Autodesk Fusion 360 part; units mm, degrees
sketch "Sketch1" plane through (0, 0, 0) normal (0, 0, 1) x (1, 0, 0)
  line L0 (0, 0) -> (50.8, 0)
  line L1 (50.8, 0) -> (50.8, 50.8)
  line L2 (50.8, 50.8) -> (0, 50.8)
  line L3 (0, 50.8) -> (0, 0)
  dimension "d1" = 50.8
  dimension "d2" = 50.8
extrude "Extrude1" add sketch "Sketch1" along normal blind 31.75
sketch "Sketch2" plane through (50.8, 0, 0) normal (1, 0, 0) x (0, 1, 0)
  line L0 (0, 0) -> (50.8, 0)
  line L1 (50.8, 0) -> (50.8, 31.75)
  line L2 (50.8, 31.75) -> (0, 31.75)
  line L3 (0, 31.75) -> (0, 0)
  line L4 (50.8, 23.368) -> (10.16, 23.368)
  line L5 (10.16, 23.368) -> (10.16, 3.81)
  line L6 (10.16, 3.81) -> (50.8, 3.81)
  line L7 (50.8, 3.81) -> (50.8, 23.368)
  dimension "d5" = 40.64
  dimension "d6" = 19.558
  dimension "d14" = 3.81
extrude "Extrude2" cut sketch "Sketch2" against normal blind 40.64 contours L1 L4 L5 L6 L7
sketch "Sketch3" plane through (0, 0, 31.75) normal (0, 0, 1) x (-1, 0, 0)
  line L0 (0, -50.8) -> (0, 0)
  line L1 (0, 0) -> (-50.8, 0)
  line L2 (-50.8, 0) -> (-50.8, -50.8)
  line L3 (-50.8, -50.8) -> (0, -50.8)
  line L4 (0, 0) -> (-25.4, 0)
  line L5 (-25.4, 0) -> (-25.4, -25.4)
  line L6 (-25.4, -25.4) -> (0, -25.4)
  line L7 (0, -25.4) -> (0, 0)
  dimension "d10" = 25.4
  dimension "d11" = 25.4
extrude "Extrude3" add sketch "Sketch3" along normal blind 152.4 contours L0 L1 L4 L5 L6 L7
fillet "Fillet1" radius 2.54 2 edges at (25.4, 12.7, 31.75) (12.7, 25.4, 31.75)
sketch "Sketch4" plane through (0, 0, 0) normal (0, 0, -1) x (1, 0, 0)
  line L0 (0, 0) -> (0, -50.8)
  line L1 (0, -50.8) -> (50.8, -50.8)
  line L2 (50.8, -50.8) -> (50.8, 0)
  line L3 (50.8, 0) -> (0, 0)
  line L4 (2.54, -2.54) -> (22.86, -2.54)
  line L5 (22.86, -2.54) -> (22.86, -22.86)
  line L6 (22.86, -22.86) -> (2.54, -22.86)
  line L7 (2.54, -22.86) -> (2.54, -2.54)
  dimension "d17" = 2.54
  dimension "d18" = 2.54
  dimension "d19" = 20.32
  dimension "d20" = 20.32
sketch "Sketch5" plane through (0, 0, 0) normal (0, 0, -1) x (1, 0, 0)
  line L0 (5.08, -5.08) -> (20.32, -5.08)
  line L1 (20.32, -5.08) -> (20.32, -20.32)
  line L2 (20.32, -20.32) -> (5.08, -20.32)
  line L3 (5.08, -20.32) -> (5.08, -5.08)
  line L4 (2.54, -2.54) -> (22.86, -2.54)
  line L5 (2.54, -22.86) -> (2.54, -2.54)
  dimension "d21" = 2.54
  dimension "d22" = 2.54
  dimension "d23" = 15.24
  dimension "d24" = 15.24
extrude "Extrude4" add sketch "Sketch5" along normal blind 2.54
loft "Loft1" add profiles "Sketch4" section 1 contours L4 L5 L6 L7 section 2 face at (10.16, 15.24, -2.54)
sketch "Sketch6" plane through (0, 0, 184.15) normal (0, 0, 1) x (-1, 0, 0)
  line L0 (0, -25.4) -> (0, 0)
  line L1 (0, 0) -> (-25.4, 0)
  line L2 (-25.4, 0) -> (-25.4, -25.4)
  line L3 (-25.4, -25.4) -> (0, -25.4)
  line L4 (-2.54, -22.86) -> (-22.86, -22.86)
  line L5 (-22.86, -22.86) -> (-22.86, -2.54)
  line L6 (-22.86, -2.54) -> (-2.54, -2.54)
  line L7 (-2.54, -2.54) -> (-2.54, -22.86)
  line L8 (-5.08, -20.32) -> (-20.32, -20.32)
  line L9 (-20.32, -20.32) -> (-20.32, -5.08)
  line L10 (-20.32, -5.08) -> (-5.08, -5.08)
  line L11 (-5.08, -5.08) -> (-5.08, -20.32)
  dimension "d27" = 2.54
  dimension "d28" = 2.54
  dimension "d29" = 2.54
  dimension "d30" = 20.32
  dimension "d31" = 2.54
  dimension "d32" = 15.24
  dimension "d33" = 15.24
  dimension "d34" = 2.54
extrude "Extrude5" cut sketch "Sketch6" against normal blind 2.54 contours L8 L9 L10 L11
loft "Loft2" cut profiles "Sketch6" section 1 contours L4 L5 L6 L7 section 2 face at (15.24, 15.24, 181.61)

Autodesk Fusion 360 part; units mm, degrees
sketch "Sketch1" plane through (0, 0, 0) normal (0, 0, 1) x (1, 0, 0)
  line L0 (0, 0) -> (1524, 0)
  line L1 (1524, 0) -> (1524, 234.95)
  line L2 (1524, 234.95) -> (0, 234.95)
  line L3 (0, 234.95) -> (0, 0)
  dimension "d1" = 234.95
  dimension "d2" = 1524
extrude "Extrude1" add sketch "Sketch1" along normal blind 19.558
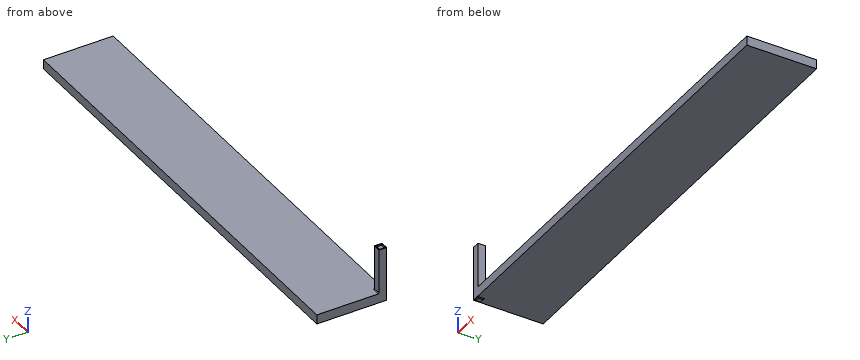
Read the model definition and answer for the solid it produces. Units are mm, in the model's axes. Round coordinates to 2 decimals unless told otherwise and drop trailing zeros. Write each loop counter-clockwise with the first axis right and the second up, starting at its lowest first coordinate (ties: lowest second). Pieces come first, ordered by that corner, then holes. Notation, with made-up numbers: (65.25, 53) -> (90.25, 53) arc R18 cw to (90.25, 75) -> close; hole circle Ø8 at (47, 18). An arc over 180 degrees is marked (long way). Answer in a Markdown table with one row per item. Add a question column.
1) Given P1, Ø12.5, axis at x = 8, z = 141.5, coming from the +Y side; P2, Ø4, axis at x = 1332.5, y = 147.5, coming from the -Z side; P3, Ø17, axis at x = 14, y = 13, coming from the +Z side, each flat-ended and moving along its own axis, determine where each tip first touches the part or whether it passes through.
2) Find section B-B, the plane x = 273. Determine the outline of the cut face in (y, z).
3) Find section A-A, the plane z = 67.5. Determine the outline of the cut face in (x, y).
4) Consider line 1 (Z direction, x = 917, y = 161). Determine where the line is inside the solid, lowest interval first.
Findings below:
| question | item | result |
|---|---|---|
| 1 | P1 | y = 25.4 |
| 1 | P2 | z = 0 |
| 1 | P3 | z = 183.79 |
| 2 | outline | (0, 0) -> (234.95, 0) -> (234.95, 31.75) -> (0, 31.75) -> close |
| 3 | outline | (0, 0) -> (25.4, 0) -> (25.4, 25.4) -> (0, 25.4) -> close |
| 4 | line 1 | 0 to 31.75 |
